```python
from build123d import *

# Parameters (mm, degrees)
CROQUIS1_R              = 10
SALIENTE_EXTRUIR1_DEPTH = 100
CROQUIS2_R              = 7.5
SALIENTE_EXTRUIR2_DEPTH = 30


with BuildPart() as part:
    # Croquis1 → Saliente-Extruir1 (new body)
    with BuildSketch(Plane.XY):
        Circle(CROQUIS1_R)
    extrude(amount=-SALIENTE_EXTRUIR1_DEPTH)

    # Croquis2 → Saliente-Extruir2 (add, symmetric)
    with BuildSketch(Plane(origin=(10, 0, 0), x_dir=(0, 0, -1), z_dir=(1, 0, 0))):
        with Locations((87.3235533, 0)):
            Circle(CROQUIS2_R)
    extrude(amount=SALIENTE_EXTRUIR2_DEPTH, both=True)


solid = part.part
```
CAD build for the part. Positions are in the model's coordinates, mm. A direction names the side the tool comes from. Round coordinates to 2 decimals unless told otherwise and drop trailing zeros. Order: outer loops, then holes, each group sorted by start corner. A loop starts at its lowest first (then second) coordinate and runs counter-clockwise, first axis right, second up. Notation, with made-up numbers: (55, 53) -> (61, 53) arc R26 ccw to (61, 86) -> close; hole circle Ø5 at (2.25, 71.25). An arc over 180 degrees is marked (long way). One line per question, with ' | ' between items.
Q1. Slice it at B-B (x = 28.5). Write the cut outline in (y, z), then the cut area to 3 significant figures.
Completed:
outline: circle Ø15 at (0, -87.32) | area: 177 mm^2
Q2. Drop flat-ended pins along their axis: pin 1 (8 mm diameter, centred on x = 6.5, z = -23.5, fed in from +Y); pin 2 (1 mm diameter, centred on y = -7, z = -70, fed in from -X); pin 3 (8 mm diameter, centred on x = 28, y = -2.5, fed in from -Z). Give the stop position or say it passes through.
Completed:
pin 1: stops at y = 9.68 | pin 2: stops at x = -7.6 | pin 3: stops at z = -94.82
Q3. Probe probe 1 along Y at (x, z) = (-0.5, -61); probe 2 along X at (y, z) = (0.25, -36); probe 3 along Z at (x, y) = (12.5, -0.5). List the from-to ranges inside material, lowest first.
Completed:
probe 1: y = -9.99 to 9.99 | probe 2: x = -10 to 10 | probe 3: z = -94.81 to -79.84
Q4. Slice it at C-C (z = -28). Write the cut outline in (x, y).
Completed:
outline: circle Ø20 at (0, 0)
Q5. Which spindle directions (+Z, -Z, +X, -X, +Y, -Y) get a long thin tool onto all of the face, cutting with end or side? Do faces 1 (the cylindrical face through (23.541, 7.436, -86.347)), 2 (the flat face through (40, 0, -87)), 3 (the cylindrical face through (-14.701, 5.069, -81.796)). Say none if no direction does.
Completed:
face 1: +X | face 2: +Z, -Z, +X, +Y, -Y | face 3: -X
Q6. Slice it at A-A (y = 0). Write the cut outline in (x, z).
Completed:
outline: (-20, -94.82) -> (-10, -94.82) -> (-10, -100) -> (10, -100) -> (10, -94.82) -> (40, -94.82) -> (40, -79.82) -> (10, -79.82) -> (10, 0) -> (-10, 0) -> (-10, -79.82) -> (-20, -79.82) -> close
Q7. Slice it at D-D (y = -6.5). Write the cut outline in (x, z).
Completed:
outline: (-20, -91.07) -> (-7.6, -91.07) -> (-7.6, -100) -> (7.6, -100) -> (7.6, -91.07) -> (40, -91.07) -> (40, -83.58) -> (7.6, -83.58) -> (7.6, 0) -> (-7.6, 0) -> (-7.6, -83.58) -> (-20, -83.58) -> close
